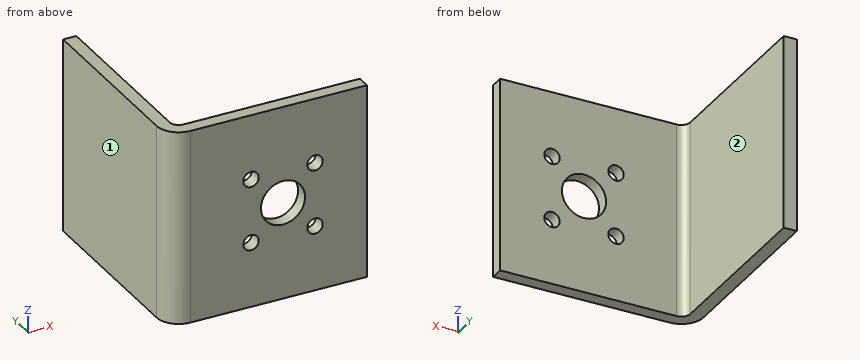
Autodesk Inventor part; units mm, degrees
ref_plane "YZ Plane" through (0, 0, 0) normal (1, 0, 0) x (0, 1, 0)
ref_plane "XZ Plane" through (0, 0, 0) normal (0, 1, 0) x (-1, 0, 0)
ref_plane "XY Plane" through (0, 0, 0) normal (0, 0, 1) x (1, 0, 0)
sketch "Sketch1" plane through (0, 0, 0) normal (0, 0, 1) x (1, 0, 0)
  line L0 (19, 0) -> (-21, 0)
  line L1 (-26, 0) -> (-26, -3)
  line L2 (-26, -3) -> (19, -3)
  line L3 (19, -3) -> (19, 0)
  line L4 (-26, -3) -> (-23, -3)
  line L5 (-23, 2) -> (-23, 42)
  line L6 (-23, 42) -> (-26, 42)
  line L7 (-26, 42) -> (-26, -3)
  arc A0 (-23, 2) -> (-21, 0) centre (-21, 2) ccw
  arc A1 (-26, 2) -> (-21, -3) centre (-21, 2) ccw
  point P0 (0, 0)
  point P1 (19, -1.5)
  dimension "d0" = 45
  dimension "d1" = 19
  dimension "d2" = 45
  dimension "d3" = 3
  dimension "d4" = 3
  dimension "d5" = 2
extrude "Extrusion1" add sketch "Sketch1" along normal mid plane 44 contours L3 L2 A1 L7 L6 L5 A0 L0
sketch "Sketch2" plane through (-21, -3, 22) normal (0, -1, 0) x (1, 0, 0)
  circle A0 centre (21, -22) radius 5
  dimension "d8" = 10
extrude "Extrusion2" cut sketch "Sketch2" against normal through all
sketch "Sketch3" plane through (-21, -3, 22) normal (0, -1, 0) x (1, 0, 0)
  point P0 (21, -22)
sketch "Sketch4" plane through (-21, -3, 22) normal (0, -1, 0) x (1, 0, 0)
  line L0 (28.25, -14.75) -> (13.75, -14.75) construction
  line L1 (13.75, -14.75) -> (13.75, -29.25) construction
  line L2 (13.75, -29.25) -> (28.25, -29.25) construction
  line L3 (28.25, -29.25) -> (28.25, -14.75) construction
  line L4 (28.25, -14.75) -> (13.75, -29.25) construction
  line L5 (13.75, -14.75) -> (28.25, -29.25) construction
  circle A0 centre (28.25, -29.25) radius 1.75
  circle A1 centre (13.75, -29.25) radius 1.75
  circle A2 centre (13.75, -14.75) radius 1.75
  circle A3 centre (28.25, -14.75) radius 1.75
  point P0 (21, -22)
  dimension "d11" = 14.5
  dimension "d12" = 14.5
  dimension "d13" = 3.5
  dimension "d14" = 3.5
  dimension "d15" = 3.5
  dimension "d16" = 3.5
extrude "Extrusion3" cut sketch "Sketch4" against normal up to surface (3 mm away)
equation "\"d14\" = d13"
equation "\"d15\" = d13"
equation "\"d16\" = d13"
properties part number "Angle_motor"
Check sheet for the modelled part. Datum: model origin and axes. Units: mm. Face numbers are marked on the shaded views. A direction names the side the tool comes from. Give positions to 0.01 mm unless a question says otherwise; leave off trailing zeros. Write each loop counter-clockwise with the first axis right and the second up, starting at its lowest first coordinate (ties: lowest second). Pieces come first, ordered by that corner, then holes. Notation, with made-up numbers: (76, 67.5) -> (119, 67.5) arc R29 cw to (119, 94.5) -> close; hole circle Ø3 at (-23.75, -0.5). An arc over 180 degrees is marked (long way). Write item = value, one per line.
Item 1: Sectioned sample at A-A on x = 0. Record the boundary of the cut face in (y, z), and give its area (3 significant figures).
Output:
outline = (-3, -22) -> (0, -22) -> (0, -5) -> (-3, -5) -> close; (-3, 5) -> (0, 5) -> (0, 22) -> (-3, 22) -> close
area = 102 mm^2
Item 2: Sectioned sample at C-C on z = 7.25. Record the boundary of the cut face in (x, y).
Output:
outline = (-26, 2) arc R5 ccw to (-21, -3) -> (-9, -3) -> (-9, 0) -> (-21, 0) arc R2 cw to (-23, 2) -> (-23, 42) -> (-26, 42) -> close; (-5.5, -3) -> (5.5, -3) -> (5.5, 0) -> (-5.5, 0) -> close; (9, -3) -> (19, -3) -> (19, 0) -> (9, 0) -> close
Item 3: Sectioned sample at B-B on z = 0. Record the boundary of the cut face in (x, y).
Output:
outline = (-26, 2) arc R5 ccw to (-21, -3) -> (-5, -3) -> (-5, 0) -> (-21, 0) arc R2 cw to (-23, 2) -> (-23, 42) -> (-26, 42) -> close; (5, -3) -> (19, -3) -> (19, 0) -> (5, 0) -> close
Item 4: Scan lines: probe 1 along Z at (x, y) = (-7.25, -0.8); probe 2 along Z at (x, y) = (0, -1); probe 3 along Y at (x, z) = (0, 9). Record each from-to range of solid material in increasing order. Write a range as from..to.
Output:
probe_1 = -22..-9, -5.5..5.5, 9..22
probe_2 = -22..-5, 5..22
probe_3 = -3..0
Item 5: Gauge pin test, flat ends, axial feed: pin 1 (1 mm diameter, centred on x = -10, z = -15.5, fed in from +Y); pin 2 (4 mm diameter, centred on y = 18.5, z = -15, fed in from +X). Record the tip position at first contact, or that the pin passes through.
Output:
pin_1 = 0
pin_2 = -23
Item 6: Tool access check on the marked faces 1 and 2. Record the directions out of +Z, -Z, +X, -X, +Y, -Y that give a thin tool (end or side, any length) a straight path to the whole face; none if there is none.
Output:
face_1 = +Z, -Z, -X, +Y, -Y
face_2 = +Z, -Z, +X, +Y
Item 7: Sectioned sample at D-D on x = 7.25. Record the boundary of the cut face in (y, z).
Output:
outline = (-3, -22) -> (0, -22) -> (0, -9) -> (-3, -9) -> close; (-3, -5.5) -> (0, -5.5) -> (0, 5.5) -> (-3, 5.5) -> close; (-3, 9) -> (0, 9) -> (0, 22) -> (-3, 22) -> close
